from build123d import *

# Parameters (mm, degrees)
F1_DEPTH = 12.7
F2_R     = 2.048268854
F2_R_2   = 1.4747920456
F3_DEPTH = 0.254


# Not quite as in the source:
# - a feature names something its author has since deleted; it is built from what else it names
# - the program builds the solid bodies; features that only make, move or delete a surface that nothing else refers to are left out


with BuildPart() as f1:
    # F0 (on Front) → F1 (new body)
    with BuildSketch(Plane.XZ):
        with BuildLine():
            Line((40.8309073806, 93.5981370211), (-25.1690926194, 93.5981370211))
            ThreePointArc((-25.1690926194, 93.5981370211), (-29.65922068, 91.7382650816), (-31.5190926194, 87.2481370211))
            Line((-31.5190926194, 87.2481370211), (-31.5190926194, -57.0518629789))
            ThreePointArc((-31.5190926194, -57.0518629789), (-29.65922068, -61.5419910395), (-25.1690926194, -63.4018629789))
            Line((-25.1690926194, -63.4018629789), (40.8309073806, -63.4018629789))
            ThreePointArc((40.8309073806, -63.4018629789), (45.3210354411, -61.5419910395), (47.1809073806, -57.0518629789))
            Line((47.1809073806, -57.0518629789), (47.1809073806, 87.2481370211))
            ThreePointArc((47.1809073806, 87.2481370211), (45.3210354411, 91.7382650816), (40.8309073806, 93.5981370211))
        make_face()
    extrude(amount=F1_DEPTH)

    # F2 (on face) → F3 (cut)
    with BuildSketch(Plane.XZ.offset(12.7)):
        with Locations((-13.1258289722, 87.2481370211)):
            Circle(F2_R)
        with Locations((0, 88.9561623335)):
            Circle(F2_R_2)
        with BuildLine():
            Line((5.0678964471, 85.2992907166), (-4.9437066773, 85.2992907166))
            ThreePointArc((-4.9437066773, 85.2992907166), (-5.2614981956, 85.1676571598), (-5.3931317525, 84.8498656414))
            Line((-5.3931317525, 84.8498656414), (-5.3931317525, 81.9237329997))
            ThreePointArc((-5.3931317525, 81.9237329997), (-5.2614981956, 81.6059414814), (-4.9437066773, 81.4743079245))
            Line((-4.9437066773, 81.4743079245), (5.0678964471, 81.4743079245))
            ThreePointArc((5.0678964471, 81.4743079245), (5.3856879655, 81.6059414814), (5.5173215223, 81.9237329997))
            Line((5.5173215223, 81.9237329997), (5.5173215223, 84.8498656414))
            ThreePointArc((5.5173215223, 84.8498656414), (5.3856879655, 85.1676571598), (5.0678964471, 85.2992907166))
        make_face()
        with BuildLine():
            Line((44.9024620466, 78.5618498921), (-28.8875750266, 78.5618498921))
            ThreePointArc((-28.8875750266, 78.5618498921), (-29.2053665449, 78.4302163352), (-29.3370001018, 78.1124248169))
            Line((-29.3370001018, 78.1124248169), (-29.3370001018, -45.495712664))
            ThreePointArc((-29.3370001018, -45.495712664), (-29.2053665449, -45.8135041823), (-28.8875750266, -45.9451377392))
            Line((-28.8875750266, -45.9451377392), (44.9024620466, -45.9451377392))
            ThreePointArc((44.9024620466, -45.9451377392), (45.2202535649, -45.8135041823), (45.3518871218, -45.495712664))
            Line((45.3518871218, -45.495712664), (45.3518871218, 78.1124248169))
            ThreePointArc((45.3518871218, 78.1124248169), (45.2202535649, 78.4302163352), (44.9024620466, 78.5618498921))
        make_face()
    extrude(amount=-F3_DEPTH, mode=Mode.SUBTRACT)


solid = f1.part
Geometry check sheet. Reference: the model listing, model coordinates, mm. A direction names the side the tool comes from. Round coordinates to 2 decimals unless told otherwise and drop trailing zeros. Order: outer loops, then holes, each group sorted by start corner. A loop starts at its lowest first (then second) coordinate and runs counter-clockwise, first axis right, second up. Notation, with made-up numbers: M 71.5,-13 L 94.5,-13 A12 ccw 94.5,1 Z; hole C 44.5,-33 d5. An arc over 180 degrees is marked long. Answer in a Markdown table with one row per item. Add a question column.
Item 1: Sectioned sample at B-B, the plane z = 69. Enter the section's corners in (x, y), plus the area to 3 significant figures.
Item 2: Draft check along Z on faces 1 (the face through (-13, -12.446, 87)), 2 (the face through (47.181, -6, 14)), 3 (the face through (45.27, -6.26, -61.59)). Enter one of: released by +Z, released by -Z, zero draft, split by the parting line, or undercut.
Item 3: Depth check by flat-ended pin: pin 1 Ø1.9 at (x, z) = (-2, 83.5) entering from -Y. Enter the tip coordinate at first touch or a pass-through.
Item 4: Sectioned sample at A-A, the plane x = 0. Enter the section's corners in (y, z), plus the area to 3 significant figures.
Item 5: Sectioned sample at C-C, the plane x = -23.5. Enter the section's corners in (y, z).
Item 6: Material ranges on L1, parallel to Z at x = 0, y = -12.55; L2, parallel to Y at x = 22.5, z = 2; L3, parallel to Z at x = 44.5, y = -4.75, recorded low to high. Write a range as [from, to].
Item 7: Set-up check for faces 4 (the face through (7, -6, -63.402)), 5 (the face through (0, -12.446, 83)): record each of +Z, -Z, +X, -X, +Y, -Y from which the full face is reachable in a straight line by a thin tool's end or side.
Filled in:
| question | item | result |
|---|---|---|
| 1 | outline | M -31.52,-12.7 L -29.34,-12.7 L -29.34,-12.45 L 45.35,-12.45 L 45.35,-12.7 L 47.18,-12.7 L 47.18,0 L -31.52,0 Z |
| 1 | area | 981 mm² |
| 2 | face 1 | undercut |
| 2 | face 2 | zero draft |
| 2 | face 3 | released by -Z |
| 3 | pin 1 | stops at y = -12.45 |
| 4 | outline | M -12.7,-63.4 L 0,-63.4 L 0,93.6 L -12.7,93.6 L -12.7,90.43 L -12.45,90.43 L -12.45,87.48 L -12.7,87.48 L -12.7,85.3 L -12.45,85.3 L -12.45,81.47 L -12.7,81.47 L -12.7,78.56 L -12.45,78.56 L -12.45,-45.95 L -12.7,-45.95 Z |
| 4 | area | 1,960 mm² |
| 5 | outline | M -12.7,-63.4 L 0,-63.4 L 0,93.6 L -12.7,93.6 L -12.7,78.56 L -12.45,78.56 L -12.45,-45.95 L -12.7,-45.95 Z |
| 6 | L1 | z = [-63.4, -45.95], [78.56, 81.47], [85.3, 87.48], [90.43, 93.6] |
| 6 | L2 | y = [-12.45, 0] |
| 6 | L3 | z = [-62.23, 92.43] |
| 7 | face 4 | -Z, +X, -X, +Y, -Y |
| 7 | face 5 | -Y |
